```python
from build123d import *

# Parameters (mm, degrees)
F1_DEPTH = 16
F2_W     = 26.482794
F2_H     = 16
F3_DEPTH = 32.841
F5_D     = 8


with BuildPart() as f1:
    # F0 (on Front) → F1 (new body, symmetric)
    with BuildSketch(Plane.XZ):
        with BuildLine():
            Line((31, 0), (0, 0))
            ThreePointArc((0, 0), (-8.455, -5.99534), (-5.594569, -15.957722))
            Line((-5.594569, -15.957722), (15.523241, -32.84))
            Line((15.523241, -32.84), (25.036241, -32.84))
            ThreePointArc((25.036241, -32.84), (30.536241, -27.34), (25.036241, -21.84))
            ThreePointArc((25.036241, -21.84), (23.536241, -20.34), (25.036241, -18.84))
            Line((25.036241, -18.84), (31, -18.84))
            ThreePointArc((31, -18.84), (40.42, -9.42), (31, 0))
        make_face()
    extrude(amount=F1_DEPTH, both=True)

    # F2 (on face) → F3 (cut, through all)
    with BuildSketch(Plane(origin=(0, 0, -32.84), x_dir=(1, 0, 0), z_dir=(0, 0, -1))):
        with Locations((4.281844, 0)):
            Rectangle(F2_W, F2_H)
    extrude(amount=-F3_DEPTH, mode=Mode.SUBTRACT)

    # F5 (through all)
    with Locations(Plane.XZ.offset(16)):
        with Locations((0, -8.959553), (31, -9.42)):
            Hole(F5_D / 2)


solid = f1.part
```
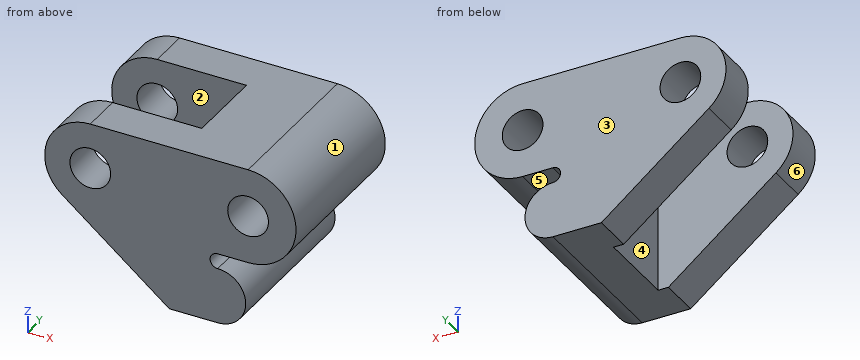
Check sheet for the modelled part. Datum: model origin and axes. Units: mm. Face numbers are marked on the shaded views. A direction names the side the tool comes from. Round coordinates to 2 decimals unless told otherwise and drop trailing zeros. Write each loop counter-clockwise with the first axis right and the second up, starting at its lowest first coordinate (ties: lowest second). Pieces come first, ordered by that corner, then holes. Notation, with made-up numbers: M -35.75,-32.75 L 13.25,-32.75 A21 ccw 13.25,2.25 Z; hole C 9.5,14.5 d7. An arc over 180 degrees is marked long. Write item = value, one per line. Start each with the question number.
1. Scan lines: line 1 (Y direction, x = 8.5, z = -2); line 2 (Z direction, x = 26, y = -5); line 3 (X direction, y = 6, z = -9). Record each from-to range of solid material in increasing order. Write a range as [from, to].
2. Gauge pin test, flat ends, axial feed: pin 1 (10 mm diameter, centred on y = 6.5, z = -12, fed in from +X); pin 2 (8 mm diameter, centred on y = -2.5, z = -19, fed in from -X); pin 3 (1.8 mm diameter, centred on x = 29.5, y = 7.5, fed in from -Z); pin 4 (10 mm diameter, centred on y = -5, z = -24, fed in from +X). Record the tip position at first contact, or that the pin passes through.
3. Tool access check on the marked faces 4, 5 and 6. Record the directions out of +Z, -Z, +X, -X, +Y, -Y that give a thin tool (end or side, any length) a straight path to the whole face; none if there is none.
4. Section check C-C, the plane y = 12. Record the cut outline in (x, z).
5. Release check for a two-part mould opening along Y. For the marked faces 1, 2 and 3 record: pulls with the +Y half, pulls with the -Y half, needs draft (parallel to the pull), parting line crosses it, or undercut.
6. Section check D-D, the plane z = -20.34. Record the cut outline in (x, y).
7. Section check B-B, the plane x = 32. Record the cut outline in (y, z), then the cut area to 3 significant figures.
8. Section check A-A, the plane y = 3.5. Record the cut outline in (x, z), then the cut area to 3 significant figures.
Results found:
q1.line_1 = [-16, -8], [8, 16]
q1.line_2 = [-32.75, -21.93], [-18.84, 0]
q1.line_3 = [17.52, 27.02], [34.98, 40.41]
q2.pin_1 = 40.42
q2.pin_2 = 17.52
q2.pin_3 = -31.53
q2.pin_4 = 30.54
q3.face_4 = +Z, -Z, -X
q3.face_5 = +X, +Y, -Y
q3.face_6 = -X, +Y, -Y
q4.outline = M -5.59,-15.96 L 15.52,-32.84 L 25.04,-32.84 A5.5 ccw 25.04,-21.84 A1.5 cw 25.04,-18.84 L 31,-18.84 A9.42 ccw 31,0 L 0,0 A8.96 ccw Z; hole C 0,-8.96 d8; hole C 31,-9.42 d8
q5.face_1 = needs draft
q5.face_2 = undercut
q5.face_3 = pulls with the +Y half
q6.outline = M -0.11,-16 L 23.54,-16 L 23.54,16 L -0.11,16 L -0.11,8 L 17.52,8 L 17.52,-8 L -0.11,-8 Z
q7.outline = M -16,-18.79 L 16,-18.79 L 16,-13.29 L -16,-13.29 Z; M -16,-5.55 L 16,-5.55 L 16,-0.05 L -16,-0.05 Z
q7.area = 352 mm^2
q8.outline = M 17.52,-32.84 L 25.04,-32.84 A5.5 ccw 25.04,-21.84 A1.5 cw 25.04,-18.84 L 31,-18.84 A9.42 ccw 31,0 L 17.52,0 Z; hole C 31,-9.42 d8
q8.area = 492 mm^2
